Verification items for the finished model (mm, model axes). A direction names the side the tool comes from. Give positions to 0.01 mm unless a question says otherwise; leave off trailing zeros. Write each loop counter-clockwise with the first axis right and the second up, starting at its lowest first coordinate (ties: lowest second). Pieces come first, ordered by that corner, then holes. Notation, with made-up numbers: M -34,58 L 5,58 A25 ccw 5,72 Z; hole C 3.5,45.25 d6. An arc over 180 degrees is marked long. Write item = value, one per line.
from build123d import *

# Parameters (mm, degrees)
CYLINDER043_R     = 1.5
CYLINDER043_DEPTH = 27
CYLINDER042_R     = 1.5
CYLINDER042_DEPTH = 27
SKETCH012_R       = 5
PAD007_DEPTH      = 30
CYLINDER029_R     = 1.5
CYLINDER029_DEPTH = 10
CYLINDER030_R     = 1.5
CYLINDER030_DEPTH = 10
CYLINDER031_R     = 1.5
CYLINDER031_DEPTH = 10
CYLINDER032_R     = 1.5
CYLINDER032_DEPTH = 11
CYLINDER033_R     = 1.5
CYLINDER033_DEPTH = 11
CYLINDER028_R     = 1.5
CYLINDER028_DEPTH = 10
BOX007_W          = 7
BOX007_H          = 15
BOX007_DEPTH      = 18
PAD006_DEPTH      = 21
BOX006_W          = 7
BOX006_H          = 15
BOX006_DEPTH      = 18
SKETCH016_R       = 2.7
SKETCH016_R_2     = 1.5
SKETCH016_R_3     = 5
SKETCH016_R_4     = 0.7
SKETCH016_W       = 12.65
SKETCH016_H       = 25
PAD009_DEPTH      = 4.8


with BuildPart() as taladro016:
    # Cylinder043 → Cylinder043 (new body)
    with BuildSketch(Plane(origin=(8.5, 26.5, -1.7), x_dir=(1, 0, 0), z_dir=(0, 0, 1))):
        Circle(CYLINDER043_R)
    extrude(amount=CYLINDER043_DEPTH)


with BuildPart() as seg_taladros_a:
    # Cylinder042 → Cylinder042 (new body)
    with BuildSketch(Plane(origin=(-8.5, 26.5, -1.7), x_dir=(1, 0, 0), z_dir=(0, 0, 1))):
        Circle(CYLINDER042_R)
    extrude(amount=CYLINDER042_DEPTH)

    # Fusion021: union Taladro016
    add(taladro016.part)


with BuildPart() as taladro_8mm:
    # Sketch012 → Pad007 (new body)
    with BuildSketch(Plane(origin=(0, 38, 3), x_dir=(1, 0, 0), z_dir=(0, -1, 0))):
        with Locations((0, 10.102227)):
            Circle(SKETCH012_R)
    extrude(amount=PAD007_DEPTH)


with BuildPart() as taladro002:
    # Cylinder029 → Cylinder029 (new body)
    with BuildSketch(Plane(origin=(-10.5, -14, 2.3), x_dir=(1, 0, 0), z_dir=(0, 0, 1))):
        Circle(CYLINDER029_R)
    extrude(amount=CYLINDER029_DEPTH)


with BuildPart() as taladro003:
    # Cylinder030 → Cylinder030 (new body)
    with BuildSketch(Plane(origin=(10.5, -5, 2.3), x_dir=(1, 0, 0), z_dir=(0, 0, 1))):
        Circle(CYLINDER030_R)
    extrude(amount=CYLINDER030_DEPTH)


with BuildPart() as taladro004:
    # Cylinder031 → Cylinder031 (new body)
    with BuildSketch(Plane(origin=(10.5, -14, 2.3), x_dir=(1, 0, 0), z_dir=(0, 0, 1))):
        Circle(CYLINDER031_R)
    extrude(amount=CYLINDER031_DEPTH)


with BuildPart() as taladro005:
    # Cylinder032 → Cylinder032 (new body)
    with BuildSketch(Plane(origin=(-8.5, 26.5, -1.7), x_dir=(1, 0, 0), z_dir=(0, 0, 1))):
        Circle(CYLINDER032_R)
    extrude(amount=CYLINDER032_DEPTH)


with BuildPart() as taladro006:
    # Cylinder033 → Cylinder033 (new body)
    with BuildSketch(Plane(origin=(8.5, 26.5, -1.7), x_dir=(1, 0, 0), z_dir=(0, 0, 1))):
        Circle(CYLINDER033_R)
    extrude(amount=CYLINDER033_DEPTH)


with BuildPart() as taladros_a:
    # Cylinder028 → Cylinder028 (new body)
    with BuildSketch(Plane(origin=(-10.5, -5, 2.3), x_dir=(1, 0, 0), z_dir=(0, 0, 1))):
        Circle(CYLINDER028_R)
    extrude(amount=CYLINDER028_DEPTH)

    # Fusion014: union Taladro002, Taladro003, Taladro004, Taladro005, Taladro006
    add(taladro002.part)
    add(taladro003.part)
    add(taladro004.part)
    add(taladro005.part)
    add(taladro006.part)


with BuildPart() as taladros_a_1:
    # Fusion014 placement: moved
    add(taladros_a.part.moved(Location((0, 0, 1))))


with BuildPart() as cubo007:
    # Box007 → Box007 (new body)
    with BuildSketch(Plane(origin=(7, -17, 3.3), x_dir=(1, 0, 0), z_dir=(0, 0, 1))):
        with Locations((3.5, 7.5)):
            Rectangle(BOX007_W, BOX007_H)
    extrude(amount=BOX007_DEPTH)


with BuildPart() as pad006:
    # Sketch011 → Pad006 (new body)
    with BuildSketch(Plane.XY.offset(-1.6)):
        Polygon((-12.559899, 30.171141), (12.559899, 30.171141), (11.070948, 23.171141), (-11.070948, 23.171141), align=None)
    extrude(amount=PAD006_DEPTH)


with BuildPart() as cut009:
    # Box006 → Box006 (new body)
    with BuildSketch(Plane(origin=(-14, -17, 3.3), x_dir=(1, 0, 0), z_dir=(0, 0, 1))):
        with Locations((3.5, 7.5)):
            Rectangle(BOX006_W, BOX006_H)
    extrude(amount=BOX006_DEPTH)

    # Fusion016: union Cubo007, Pad006
    add(cubo007.part)
    add(pad006.part)

    # Cut007: cut Taladros A
    add(taladros_a_1.part, mode=Mode.SUBTRACT)

    # Cut009: cut Taladro 8mm
    add(taladro_8mm.part, mode=Mode.SUBTRACT)


with BuildPart() as cut010:
    # Sketch016 → Pad009 (new body)
    with BuildSketch(Plane.XY.offset(19)):
        with BuildLine():
            Line((-29.572856, 5.202237), (-9, 13.39959))
            Line((-9, 13.39959), (-12.540941, 30.154421))
            Line((-12.540941, 30.154421), (12.540941, 30.154421))
            Line((9, 13.39959), (12.540941, 30.154421))
            Line((9, 13.39959), (29.570667, 5.203109))
            ThreePointArc((29.587798, -5.196258), (33.099992, 0.009225), (29.570667, 5.203109))
            Line((29.587798, -5.196258), (15.980248, -10.663617))
            ThreePointArc((15.980248, -10.663617), (14.613214, -11.767355), (14.098711, -13.447327))
            Line((14.098711, -13.447327), (14.098711, -18.900571))
            ThreePointArc((9.098711, -23.900571), (12.634245, -22.436105), (14.098711, -18.900571))
            Line((9.098711, -23.900571), (-9.098711, -23.900571))
            ThreePointArc((-14.098711, -18.900571), (-12.634245, -22.436105), (-9.098711, -23.900571))
            Line((-14.098711, -18.900571), (-14.098711, -13.447327))
            ThreePointArc((-14.098711, -13.447327), (-14.613214, -11.767355), (-15.980248, -10.663617))
            Line((-15.980248, -10.663617), (-29.587798, -5.196258))
            ThreePointArc((-29.572856, 5.202237), (-33.099994, 0.008047), (-29.587798, -5.196258))
        make_face()
        with Locations((27.5, 0)):
            Circle(SKETCH016_R, mode=Mode.SUBTRACT)
        with Locations((-27.5, 0)):
            Circle(SKETCH016_R, mode=Mode.SUBTRACT)
        with Locations((10.65, -20.334303)):
            Circle(SKETCH016_R_2, mode=Mode.SUBTRACT)
        with Locations((-10.65, -20.334303)):
            Circle(SKETCH016_R_2, mode=Mode.SUBTRACT)
        with Locations((13, 8.886284)):
            Circle(SKETCH016_R_2, mode=Mode.SUBTRACT)
        with Locations((-13, 8.886284)):
            Circle(SKETCH016_R_2, mode=Mode.SUBTRACT)
        with Locations((7.5, 20.154421)):
            Circle(SKETCH016_R_2, mode=Mode.SUBTRACT)
        with Locations((-7.5, 20.154421)):
            Circle(SKETCH016_R_2, mode=Mode.SUBTRACT)
        with Locations((0, 17.333948)):
            Circle(SKETCH016_R_3, mode=Mode.SUBTRACT)
        with Locations((0, 8.318832)):
            Circle(SKETCH016_R_4, mode=Mode.SUBTRACT)
        with Locations((0, -18.804168)):
            Circle(SKETCH016_R_4, mode=Mode.SUBTRACT)
        with Locations((0, -5.238349)):
            Rectangle(SKETCH016_W, SKETCH016_H, mode=Mode.SUBTRACT)
    extrude(amount=PAD009_DEPTH)

    # Fusion020: union Cut009
    add(cut009.part)

    # Cut010: cut Seg taladros A
    add(seg_taladros_a.part, mode=Mode.SUBTRACT)


solid = cut010.part
1) Tool access check on faces 1 (the flat face through (-11, -5, 13.3)), 2 (the flat face through (14.099, -16, 21)), 3 (the flat face through (7, -10, 11)), 4 (the flat face through (0, 23.171, 6)). Record the directions out of +Z, -Z, +X, -X, +Y, -Y that give a thin tool (end or side, any length) a straight path to the whole face; none if there is none.
From the geometry:
face_1 = -Z
face_2 = +Z, -Z, +X, -Y
face_3 = -Z, -Y
face_4 = -Z, +X, -X
2) Material ranges on probe 1 along X at (y, z) = (-10, 8.75); probe 2 along Y at (x, z) = (7.5, 21.65); probe 3 along Y at (x, z) = (-7.5, 9), recorded low to high. Write a range as from..to.
From the geometry:
probe_1 = -14..-7, 7..14
probe_2 = -23.9..18.65, 21.65..25.38, 27.62..30.15
probe_3 = -17..-2, 23.17..25.38, 27.62..30.17
3) Cross-section at A-A on z = 5.25. Count the separate pieces of the cut face and the enclosed holes in it, plus the area to 3 significant figures.
From the geometry:
separate_pieces = 3
enclosed_holes = 6
area = 333 mm^2
4) Cross-section at D-D on x = -27.5. Record the boundary of the cut face in (y, z).
From the geometry:
outline = M -6.04,19 L -2.7,19 L -2.7,23.8 L -6.04,23.8 Z; M 2.7,19 L 6.03,19 L 6.03,23.8 L 2.7,23.8 Z
5) Depth check by flat-ended pin: P1, Ø8, axis at x = 25.5, y = 4.5, coming from the -Z side; P2, Ø2.5, axis at x = -8.5, y = 26.5, coming from the -Z side; P3, Ø2, axis at x = -9.5, y = -10.5, coming from the -Z side; P4, Ø7.5, axis at y = -12, z = 9.5, coming from the +X side. Enter the tip coordinate at first touch or a pass-through.
From the geometry:
P1 = 19
P2 = through
P3 = 3.3
P4 = 14
6) Draft check along X on faces 5 (the cylindrical face through (33.1, -0.1, 21.4)), 6 (the flat face through (0, -23.901, 21)), 7 (the cylindrical face through (-0.152, -19.488, 21.366)). Enter one of: +X half, -X half, draft (parallel to the pull), parting line (faces both ways), or undercut.
From the geometry:
face_5 = +X half
face_6 = draft
face_7 = undercut
